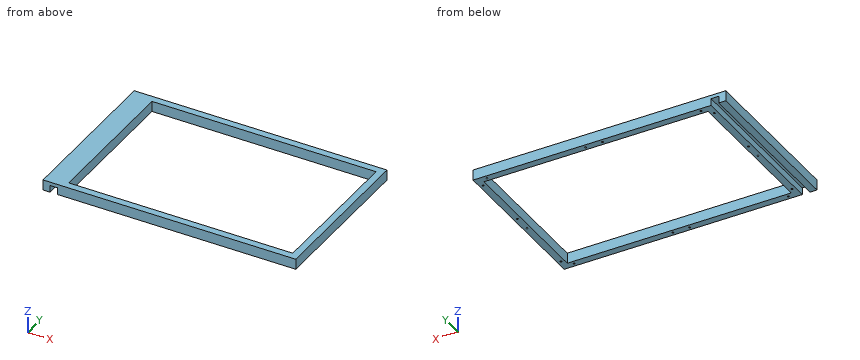
```python
from build123d import *

# Parameters (mm, degrees)
CYLINDER047_R     = 1.3
CYLINDER047_DEPTH = 146
CYLINDER045_R     = 1.3
CYLINDER045_DEPTH = 146
CYLINDER043_R     = 1.3
CYLINDER043_DEPTH = 146
CYLINDER040_R     = 1.3
CYLINDER040_DEPTH = 146
CYLINDER039_R     = 1.3
CYLINDER039_DEPTH = 146
CYLINDER036_R     = 1.3
CYLINDER036_DEPTH = 146
CYLINDER034_R     = 1.3
CYLINDER034_DEPTH = 146
CYLINDER032_R     = 1.3
CYLINDER032_DEPTH = 146
CYLINDER030_R     = 1.3
CYLINDER030_DEPTH = 146
CYLINDER018_R     = 1.3
CYLINDER018_DEPTH = 146
CYLINDER017_R     = 1.3
CYLINDER017_DEPTH = 146
CYLINDER012_R     = 1.3
CYLINDER012_DEPTH = 146
CYLINDER011_R     = 1.3
CYLINDER011_DEPTH = 146
CYLINDER009_R     = 1.3
CYLINDER009_DEPTH = 146
CYLINDER002_R     = 1.3
CYLINDER002_DEPTH = 146
CYLINDER001_R     = 1.3
CYLINDER001_DEPTH = 146
BOX046_W          = 10
BOX046_H          = 230
BOX046_DEPTH      = 10
BOX041_W          = 10
BOX041_H          = 210
BOX041_DEPTH      = 15
BOX040_W          = 340
BOX040_H          = 10
BOX040_DEPTH      = 15
BOX024_W          = 10
BOX024_H          = 210
BOX024_DEPTH      = 15
BOX042_W          = 340
BOX042_H          = 10
BOX042_DEPTH      = 15
BOX045_W          = 21
BOX045_H          = 230
BOX045_DEPTH      = 5


with BuildPart() as cilindro047:
    # Cylinder047 → Cylinder047 (new body)
    with BuildSketch(Plane(origin=(5, 103, 8), x_dir=(1, 0, 0), z_dir=(0, 0, 1))):
        Circle(CYLINDER047_R)
    extrude(amount=CYLINDER047_DEPTH)


with BuildPart() as cilindro045:
    # Cylinder045 → Cylinder045 (new body)
    with BuildSketch(Plane(origin=(5, 127, 8), x_dir=(1, 0, 0), z_dir=(0, 0, 1))):
        Circle(CYLINDER045_R)
    extrude(amount=CYLINDER045_DEPTH)


with BuildPart() as cilindro043:
    # Cylinder043 → Cylinder043 (new body)
    with BuildSketch(Plane(origin=(5, 213, 8), x_dir=(1, 0, 0), z_dir=(0, 0, 1))):
        Circle(CYLINDER043_R)
    extrude(amount=CYLINDER043_DEPTH)


with BuildPart() as cilindro040:
    # Cylinder040 → Cylinder040 (new body)
    with BuildSketch(Plane(origin=(17, 225, 8), x_dir=(1, 0, 0), z_dir=(0, 0, 1))):
        Circle(CYLINDER040_R)
    extrude(amount=CYLINDER040_DEPTH)


with BuildPart() as cilindro039:
    # Cylinder039 → Cylinder039 (new body)
    with BuildSketch(Plane(origin=(158, 225, 8), x_dir=(1, 0, 0), z_dir=(0, 0, 1))):
        Circle(CYLINDER039_R)
    extrude(amount=CYLINDER039_DEPTH)


with BuildPart() as cilindro036:
    # Cylinder036 → Cylinder036 (new body)
    with BuildSketch(Plane(origin=(182, 225, 8), x_dir=(1, 0, 0), z_dir=(0, 0, 1))):
        Circle(CYLINDER036_R)
    extrude(amount=CYLINDER036_DEPTH)


with BuildPart() as cilindro034:
    # Cylinder034 → Cylinder034 (new body)
    with BuildSketch(Plane(origin=(323, 225, 8), x_dir=(1, 0, 0), z_dir=(0, 0, 1))):
        Circle(CYLINDER034_R)
    extrude(amount=CYLINDER034_DEPTH)


with BuildPart() as cilindro032:
    # Cylinder032 → Cylinder032 (new body)
    with BuildSketch(Plane(origin=(335, 213, 8), x_dir=(1, 0, 0), z_dir=(0, 0, 1))):
        Circle(CYLINDER032_R)
    extrude(amount=CYLINDER032_DEPTH)


with BuildPart() as cilindro030:
    # Cylinder030 → Cylinder030 (new body)
    with BuildSketch(Plane(origin=(335, 127, 8), x_dir=(1, 0, 0), z_dir=(0, 0, 1))):
        Circle(CYLINDER030_R)
    extrude(amount=CYLINDER030_DEPTH)


with BuildPart() as cilindro018:
    # Cylinder018 → Cylinder018 (new body)
    with BuildSketch(Plane(origin=(335, 103, 8), x_dir=(1, 0, 0), z_dir=(0, 0, 1))):
        Circle(CYLINDER018_R)
    extrude(amount=CYLINDER018_DEPTH)


with BuildPart() as cilindro017:
    # Cylinder017 → Cylinder017 (new body)
    with BuildSketch(Plane(origin=(335, 17, 8), x_dir=(1, 0, 0), z_dir=(0, 0, 1))):
        Circle(CYLINDER017_R)
    extrude(amount=CYLINDER017_DEPTH)


with BuildPart() as cilindro012:
    # Cylinder012 → Cylinder012 (new body)
    with BuildSketch(Plane(origin=(323, 5, 8), x_dir=(1, 0, 0), z_dir=(0, 0, 1))):
        Circle(CYLINDER012_R)
    extrude(amount=CYLINDER012_DEPTH)


with BuildPart() as cilindro011:
    # Cylinder011 → Cylinder011 (new body)
    with BuildSketch(Plane(origin=(182, 5, 8), x_dir=(1, 0, 0), z_dir=(0, 0, 1))):
        Circle(CYLINDER011_R)
    extrude(amount=CYLINDER011_DEPTH)


with BuildPart() as cilindro009:
    # Cylinder009 → Cylinder009 (new body)
    with BuildSketch(Plane(origin=(158, 5, 8), x_dir=(1, 0, 0), z_dir=(0, 0, 1))):
        Circle(CYLINDER009_R)
    extrude(amount=CYLINDER009_DEPTH)


with BuildPart() as cilindro002:
    # Cylinder002 → Cylinder002 (new body)
    with BuildSketch(Plane(origin=(5, 17, 8), x_dir=(1, 0, 0), z_dir=(0, 0, 1))):
        Circle(CYLINDER002_R)
    extrude(amount=CYLINDER002_DEPTH)


with BuildPart() as cilindro001:
    # Cylinder001 → Cylinder001 (new body)
    with BuildSketch(Plane(origin=(17, 5, 8), x_dir=(1, 0, 0), z_dir=(0, 0, 1))):
        Circle(CYLINDER001_R)
    extrude(amount=CYLINDER001_DEPTH)


with BuildPart() as cubo009:
    # Box046 → Box046 (new body)
    with BuildSketch(Plane(origin=(-21, 249, 0), x_dir=(1, 0, 0), z_dir=(0, 0, 1))):
        with Locations((5, 115)):
            Rectangle(BOX046_W, BOX046_H)
    extrude(amount=BOX046_DEPTH)


with BuildPart() as cubo004:
    # Box041 → Box041 (new body)
    with BuildSketch(Plane(origin=(330, 259, 0), x_dir=(1, 0, 0), z_dir=(0, 0, 1))):
        with Locations((5, 105)):
            Rectangle(BOX041_W, BOX041_H)
    extrude(amount=BOX041_DEPTH)


with BuildPart() as cubo003:
    # Box040 → Box040 (new body)
    with BuildSketch(Plane(origin=(0, 249, 0), x_dir=(1, 0, 0), z_dir=(0, 0, 1))):
        with Locations((170, 5)):
            Rectangle(BOX040_W, BOX040_H)
    extrude(amount=BOX040_DEPTH)


with BuildPart() as cubo002:
    # Box024 → Box024 (new body)
    with BuildSketch(Plane(origin=(0, 259, 0), x_dir=(1, 0, 0), z_dir=(0, 0, 1))):
        with Locations((5, 105)):
            Rectangle(BOX024_W, BOX024_H)
    extrude(amount=BOX024_DEPTH)


with BuildPart() as obj1:
    # Box042 → Box042 (new body)
    with BuildSketch(Plane(origin=(0, 469, 0), x_dir=(1, 0, 0), z_dir=(0, 0, 1))):
        with Locations((170, 5)):
            Rectangle(BOX042_W, BOX042_H)
    extrude(amount=BOX042_DEPTH)

    # Fusion004: union Cubo004, Cubo003, Cubo002
    add(cubo004.part)
    add(cubo003.part)
    add(cubo002.part)


with BuildPart() as cut062:
    # Box045 → Box045 (new body)
    with BuildSketch(Plane(origin=(-21, 249, 10), x_dir=(1, 0, 0), z_dir=(0, 0, 1))):
        with Locations((10.5, 115)):
            Rectangle(BOX045_W, BOX045_H)
    extrude(amount=BOX045_DEPTH)

    # Fusion005: union Cubo009, obj1
    add(cubo009.part)
    add(obj1.part)


with BuildPart() as cut062_1:
    # Fusion005 placement: moved
    add(cut062.part.moved(Location((0, -249, 147))))

    # Cut016: cut Cilindro001
    add(cilindro001.part, mode=Mode.SUBTRACT)

    # Cut017: cut Cilindro002
    add(cilindro002.part, mode=Mode.SUBTRACT)

    # Cut023: cut Cilindro009
    add(cilindro009.part, mode=Mode.SUBTRACT)

    # Cut026: cut Cilindro011
    add(cilindro011.part, mode=Mode.SUBTRACT)

    # Cut029: cut Cilindro012
    add(cilindro012.part, mode=Mode.SUBTRACT)

    # Cut032: cut Cilindro017
    add(cilindro017.part, mode=Mode.SUBTRACT)

    # Cut043: cut Cilindro018
    add(cilindro018.part, mode=Mode.SUBTRACT)

    # Cut045: cut Cilindro030
    add(cilindro030.part, mode=Mode.SUBTRACT)

    # Cut047: cut Cilindro032
    add(cilindro032.part, mode=Mode.SUBTRACT)

    # Cut049: cut Cilindro034
    add(cilindro034.part, mode=Mode.SUBTRACT)

    # Cut051: cut Cilindro036
    add(cilindro036.part, mode=Mode.SUBTRACT)

    # Cut054: cut Cilindro039
    add(cilindro039.part, mode=Mode.SUBTRACT)

    # Cut055: cut Cilindro040
    add(cilindro040.part, mode=Mode.SUBTRACT)

    # Cut058: cut Cilindro043
    add(cilindro043.part, mode=Mode.SUBTRACT)

    # Cut060: cut Cilindro045
    add(cilindro045.part, mode=Mode.SUBTRACT)

    # Cut062: cut Cilindro047
    add(cilindro047.part, mode=Mode.SUBTRACT)


solid = cut062_1.part
```
Build history of the part. All positions in model axes, mm. Give positions to 0.01 mm unless a question says otherwise; leave off trailing zeros. Loops run counter-clockwise (first coordinate to the right, second up) from the corner with the lowest first, then second, coordinate; pieces in that order, holes last.
1) Drop flat-ended pins along their axis: P1, Ø0.8, axis at x = 322.5, y = 224.5, coming from the -Z side; P2, Ø6, axis at x = 215, z = 150.5, coming from the -Y side. Give the stop position or say it passes through.
Values follow:
P1: stops at z = 154
P2: stops at y = 0
2) Band-saw the part on A-A on z = 150. State how many separate pieces and enclosed holes the cut face has, then the cut area to 3 significant figures.
Values follow:
separate pieces: 2
enclosed holes: 17
area: 13,200 mm2
3) Band-saw the part on C-C on x = 189.5. List the corners of the cut face in (y, z), then the cut area to 3 significant figures.
Values follow:
outline: (0, 147) - (10, 147) - (10, 162) - (0, 162) - close; (220, 147) - (230, 147) - (230, 162) - (220, 162) - close
area: 300 mm2
4) Band-saw the part on B-B on y = 33.5. List the corners of the cut face in (x, z), then the cut area to 3 significant figures.
Values follow:
outline: (-21, 147) - (-11, 147) - (-11, 157) - (0, 157) - (0, 147) - (10, 147) - (10, 162) - (-21, 162) - close; (330, 147) - (340, 147) - (340, 162) - (330, 162) - close
area: 505 mm2
5) Probe line 1 along X through (y, z) = (17, 149.5); line 2 along X through (y, z) = (129.5, 156); line 3 along Y through (x, z) = (105, 160.5). List the from-to ranges inside material, lowest first.
Values follow:
line 1: x = -21 to -11, 0 to 3.7, 6.3 to 10, 330 to 333.7, 336.3 to 340
line 2: x = -21 to -11, 0 to 10, 330 to 340
line 3: y = 0 to 10, 220 to 230
